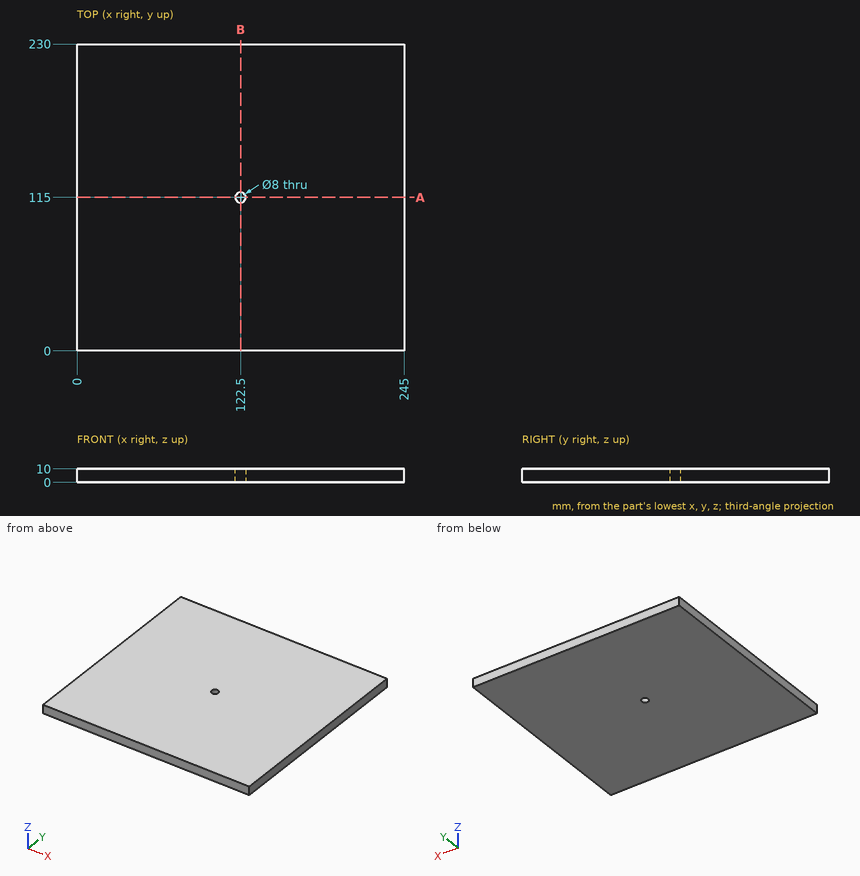
Here's the drawing with two shaded views (mm, measured from the low corner). I have some questions. Give positions to 0.01 mm unless a question says otherwise; leave off trailing zeros. Write each loop counter-clockwise with the first axis right and the second up, starting at its lowest first coordinate (ties: lowest second). Pieces come first, ordered by that corner, then holes. Notation, with made-up numbers: (12.5, -20) -> (67.5, -20) arc R28 ccw to (67.5, 10) -> close; hole circle Ø2 at (69.25, 56). An arc over 180 degrees is marked (long way). Use one line per item in the form item = value. Start each with the question number.
1. Imagine slicing it at A-A on y = 115. List the corners of the cut face in (x, z) for me, plus the area to 3 significant figures.
2. Will these pins go through, and if not, where does the flat tip stop? pin 1 Ø3 at (x, y) = (44.5, 204.5) entering from -Z; pin 2 Ø5 at (x, y) = (122.5, 115) entering from +Z.
3. If I drill on L1, parallel to Y at x = 122.5, z = 5.5, over which ranges is the centre line in solid material (lowest first)?
4. Imagine slicing it at B-B on x = 122.5. List the corners of the cut face in (y, z) for me, plus the area to 3 significant figures.
Entries:
q1.outline = (0, 0) -> (118.5, 0) -> (118.5, 10) -> (0, 10) -> close; (126.5, 0) -> (245, 0) -> (245, 10) -> (126.5, 10) -> close
q1.area = 2,370 mm²
q2.pin_1 = 0
q2.pin_2 = through
q3.L1 = 0 to 111, 119 to 230
q4.outline = (0, 0) -> (111, 0) -> (111, 10) -> (0, 10) -> close; (119, 0) -> (230, 0) -> (230, 10) -> (119, 10) -> close
q4.area = 2,220 mm²
